Read the model definition and answer for the solid it produces. Units are mm, in the model's axes. A direction names the side the tool comes from. Round coordinates to 2 decimals unless told otherwise and drop trailing zeros. Write each loop counter-clockwise with the first axis right and the second up, starting at its lowest first coordinate (ties: lowest second). Pieces come first, ordered by that corner, then holes. Notation, with made-up numbers: (79.25, 86) - (111.25, 86) arc R19 cw to (111.25, 93) - close; hole circle Ø6 at (68, -11). An arc over 180 degrees is marked (long way). Use one line per item in the form item = value. Start each with the question number.
1) The part is cut by section B-B, the plane z = 32. Give the vertices of the cut face in (x, y).
2) The part is cut by section C-C, the plane y = 25. Give the vertices of the cut face in (x, z), plus the area to 3 significant figures.
3) Consider line 1 along X through (y, z) = (12.5, 0); line 2 along Z through (x, y) = (0, 13); line 3 along Y through (x, z) = (6, -3.5). Determine where each line is inside the solid, lowest interval first. Write a range as from..to.
4) The part is cut by section A-A, the plane x = 0. Give the vertices of the cut face in (y, z), plus the area to 3 significant figures.
5) For faces 5 (the face through (2, 0, 2)), 6 (the face through (-65, 10, 2)), determine the directions among +Z, -Z, +X, -X, +Y, -Y from which every point of the face is accessible in a straight line to the end or side of a thin tool.
6) Each of these flat-tipped pins is pushed along its axis until it touches: pin 1 (10 mm diameter, centred on y = 19, z = -15, fed in from +X); pin 2 (10 mm diameter, centred on x = -28, y = 37.5, fed in from +Z); pin 3 (4 mm diameter, centred on x = -108.5, z = -91.5, fed in from +Y). Where does it stop, or does it pass through?
7) The part is cut by section D-D, the plane x = 125.5. Give the vertices of the cut face in (y, z).
8) For a pull along Z with two mould halves and no side action, classify faces 1 (the face through (59.94, 13.94, -2.64)), 2 (the face through (1, 10, 1)), 3 (the face through (-47.69, 13.94, -15.02)), 4 (the face through (23, 18, 45)) as released by +Z, released by -Z, zero draft, split by the parting line, or undercut.
Autodesk Inventor part; units mm, degrees
ref_plane "YZ Plane" through (0, 0, 0) normal (1, 0, 0) x (0, 1, 0)
ref_plane "XZ Plane" through (0, 0, 0) normal (0, 1, 0) x (-1, 0, 0)
ref_plane "XY Plane" through (0, 0, 0) normal (0, 0, 1) x (1, 0, 0)
sketch "Sketch1" plane through (0, 0, 0) normal (0, 1, 0) x (-1, 0, 0)
  line L0 (150, 150) -> (-150, 150)
  line L1 (-150, 150) -> (-150, -150)
  line L2 (-150, -150) -> (150, -150)
  line L3 (150, -150) -> (150, 150)
  circle A0 centre (0, 0) radius 50
  circle A1 centre (20, 0) radius 1.5
  circle A2 centre (0, 0) radius 60
  dimension "d0" = 100
  dimension "d1" = 300
  dimension "d2" = 300
  dimension "d3" = 150
  dimension "d4" = 150
  dimension "d5" = 3
  dimension "d6" = 20
  dimension "d11" = 120
extrude "Extrusion1" add sketch "Sketch1" along normal blind 10 contours L3 L2 L1 L0 | A0 | A1 | A2
extrude "Extrusion2" add sketch "Sketch1" along normal blind 50 contours A1
extrude "Extrusion3" add sketch "Sketch1" along normal blind 18 contours A2
properties part number "bottom-plate" material "Concrete"
Geometry results:
q1.outline = (-150, 0) - (150, 0) - (150, 10) - (50.75, 10) - (50.75, 18) - (38.42, 18) - (38.42, 10) - (-38.42, 10) - (-38.42, 18) - (-50.75, 18) - (-50.75, 10) - (-150, 10) - close
q2.outline = circle Ø3 at (-20, 0)
q2.area = 7.07 mm2
q3.line_1 = -60..-50, -21.5..-18.5, 50..60
q3.line_2 = -60..-50, 50..60
q3.line_3 = 0..10
q4.outline = (0, -150) - (10, -150) - (10, -60) - (18, -60) - (18, -50) - (10, -50) - (10, 50) - (18, 50) - (18, 60) - (10, 60) - (10, 150) - (0, 150) - close
q4.area = 3,160 mm2
q5.face_5 = +Z, -Z, +X, -X, -Y
q5.face_6 = +Y
q6.pin_1 = 59.14
q6.pin_2 = through
q6.pin_3 = 10
q7.outline = (0, -150) - (10, -150) - (10, 150) - (0, 150) - close
q8.face_1 = split by the parting line
q8.face_2 = undercut
q8.face_3 = undercut
q8.face_4 = zero draft
